Check sheet for the drawn part. Datum: minimum x, y, z corner. Units: mm. A direction names the side the tool comes from. Round coordinates to 2 decimals unless told otherwise and drop trailing zeros. Write each loop counter-clockwise with the first axis right and the second up, starting at its lowest first coordinate (ties: lowest second). Pieces come first, ordered by that corner, then holes. Notation, with made-up numbers: (51, -20) - (60, -20) arc R14 ccw to (60, -7) - close; hole circle Ø10 at (80, 34.5). An arc over 180 degrees is marked (long way). Return JSON: item names as keys, results as strings. Group by question number.
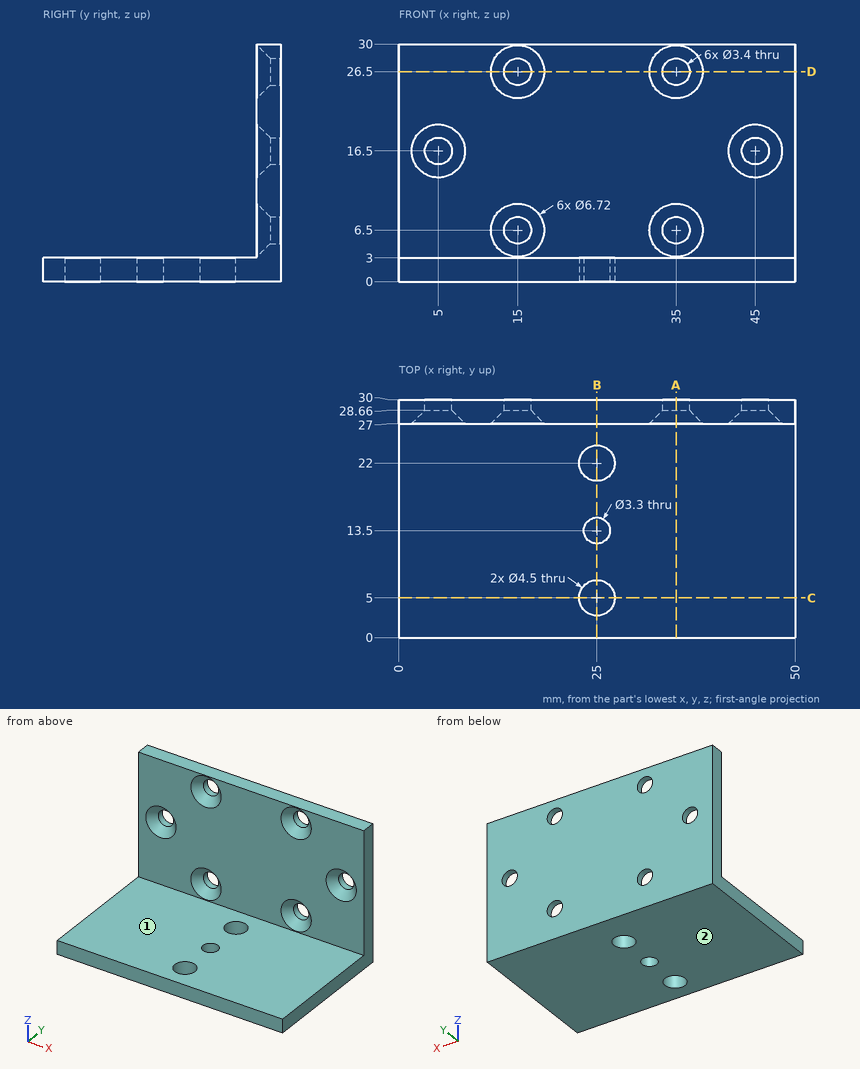
1. Section check B-B (x = 25). Enter the section's corners in (y, z).
2. Section check A-A (x = 35). Enter the section's corners in (y, z), and give its area (3 significant figures).
3. Section check C-C (y = 5). Enter the section's corners in (x, z).
4. Depth check by flat-ended pin: pin 1 Ø12 at (y, z) = (17, 25) entering from +X; pin 2 Ø5.5 at (x, z) = (15, 6.5) entering from -Y; pin 3 Ø4 at (x, z) = (35, 26.5) entering from -Y; pin 4 Ø13.5 at (x, z) = (27, 17.5) entering from -Y. Enter the tip coordinate at first touch or a pass-through.
5. Material ranges on line 1 along X through (y, z) = (28.9, 16.5); line 2 along X through (y, z) = (28.9, 6.5); line 3 along Z through (x, y) = (35, 29.1), recorded low to high.
6. Section check D-D (z = 26.5). Enter the section's corners in (x, y).
7. Tool access check on the marked faces 1 and 2. Record the directions out of +Z, -Z, +X, -X, +Y, -Y that give a thin tool (end or side, any length) a straight path to the whole face; none if there is none.
Result sheet:
{
 "1": {"outline": "(0, 0) - (2.75, 0) - (2.75, 3) - (0, 3) - close; (7.25, 0) - (11.85, 0) - (11.85, 3) - (7.25, 3) - close; (15.15, 0) - (19.75, 0) - (19.75, 3) - (15.15, 3) - close; (24.25, 0) - (30, 0) - (30, 30) - (27, 30) - (27, 3) - (24.25, 3) - close"},
 "2": {"outline": "(0, 0) - (30, 0) - (30, 4.8) - (28.66, 4.8) - (27, 3.14) - (27, 3) - (0, 3) - close; (27, 9.86) - (28.66, 8.2) - (30, 8.2) - (30, 24.8) - (28.66, 24.8) - (27, 23.14) - close; (27, 29.86) - (28.66, 28.2) - (30, 28.2) - (30, 30) - (27, 30) - close", "area": "145 mm²"},
 "3": {"outline": "(0, 0) - (22.75, 0) - (22.75, 3) - (0, 3) - close; (27.25, 0) - (50, 0) - (50, 3) - (27.25, 3) - close"},
 "4": {"pin 1": "passes through", "pin 2": "stops at y = 27.61", "pin 3": "stops at y = 28.36", "pin 4": "stops at y = 27"},
 "5": {"line 1": "x = 0 to 3.3, 6.7 to 43.3, 46.7 to 50", "line 2": "x = 0 to 13.3, 16.7 to 33.3, 36.7 to 50", "line 3": "z = 0 to 4.8, 8.2 to 24.8, 28.2 to 30"},
 "6": {"outline": "(0, 27) - (11.64, 27) - (13.3, 28.66) - (13.3, 30) - (0, 30) - close; (16.7, 28.66) - (18.36, 27) - (31.64, 27) - (33.3, 28.66) - (33.3, 30) - (16.7, 30) - close; (36.7, 28.66) - (38.36, 27) - (50, 27) - (50, 30) - (36.7, 30) - close"},
 "7": {"face 1": "+Z, +X, -X, -Y", "face 2": "-Z, +X, -X, +Y, -Y"}
}
